Build history of the part. All positions in model axes, mm. Face numbers are marked on the shaded views. A direction names the side the tool comes from. Give positions to 0.01 mm unless a question says otherwise; leave off trailing zeros. Write each loop counter-clockwise with the first axis right and the second up, starting at its lowest first coordinate (ties: lowest second). Pieces come first, ordered by that corner, then holes. Notation, with made-up numbers: (12.25, 71) -> (31.25, 71) arc R31 ccw to (31.25, 101) -> close; hole circle Ø7 at (7.25, 64.5). An arc over 180 degrees is marked (long way). Write item = value, one per line. Start each with the question number.
Q1. Wall check: line 1 (Y direction, x = -0.25, z = 3.5); line 2 (Y direction, x = -0.5, z = -0.25); line 3 (X direction, y = -3.5, z = 0.75). Give the ranges that are in metal, low to high.
Q2. Tool access for the marked faces 1, 2 and 3: list every direction of +Z, -Z, +X, -X, +Y, -Y with a clear straight run to the whole face (end or side of a thin tool).
Q3. Saw through at B-B, the plane y = 4. List the corners of the cut face in (x, z), then the cut area to 3 significant figures.
Q4. Saw through at A-A, the plane z = 0. List the corners of the cut face in (x, y).
Q5. Drop flat-ended pins along their axis: P1, Ø0.7, axis at y = -3.5, z = -0.5, coming from the -X side; P2, Ø1, axis at x = -1, y = 17, coming from the +Z side; P3, Ø2, axis at y = 10, z = 0.5, coming from the -X side. Give the stop position or say it passes through.
from build123d import *

# Parameters (mm, degrees)
F0_R     = 4.25
F1_DEPTH = 5
F2_R     = 2.1
F3_DEPTH = 22
F5_DEPTH = 2.5
F6_SIZE  = 0.4


with BuildPart() as f1:
    # F0 (on Front) → F1 (new body)
    with BuildSketch(Plane.XZ):
        Circle(F0_R)
    extrude(amount=F1_DEPTH)

    # F2 (on face) → F3 (join)
    with BuildSketch(Plane(origin=(0, 0, 0), x_dir=(-1, 0, 0), z_dir=(0, 1, 0))):
        Circle(F2_R)
    extrude(amount=F3_DEPTH)

    # F4 (on face) → F5 (cut)
    with BuildSketch(Plane.XZ.offset(5)):
        Polygon((0, -2.309401), (2, -1.154701), (2, 1.154701), (0, 2.309401), (-2, 1.154701), (-2, -1.154701), align=None)
    extrude(amount=-F5_DEPTH, mode=Mode.SUBTRACT)

    # F6
    f6_edges = [f1.edges().sort_by_distance(p)[0] for p in [
        (-4.25, -5, 0),
    ]]
    chamfer(f6_edges, length=F6_SIZE)


solid = f1.part
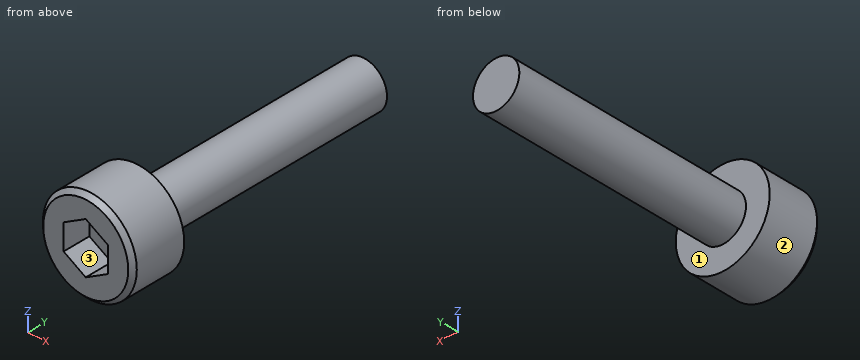
Report:
q1.line_1 = -5 to 0
q1.line_2 = -2.5 to 22
q1.line_3 = -4.18 to -2, 2 to 4.18
q2.face_1 = +Y
q2.face_2 = +Y, -Y
q2.face_3 = -Y
q3.outline = circle Ø4.2 at (0, 0)
q3.area = 13.9 mm2
q4.outline = (-4.25, -4.6) -> (-3.85, -5) -> (-2, -5) -> (-2, -2.5) -> (2, -2.5) -> (2, -5) -> (3.85, -5) -> (4.25, -4.6) -> (4.25, 0) -> (2.1, 0) -> (2.1, 22) -> (-2.1, 22) -> (-2.1, 0) -> (-4.25, 0) -> close
q5.P1 = -4.25
q5.P2 = 2.04
q5.P3 = -2.1
